Input: dimensioned drawing with shaded views. Units: mm. Origin: part minimum x, y, z. A direction names the side the tool comes from. Give positions to 0.01 mm unless a question says otherwise; leave off trailing zeros. Write each loop counter-clockwise with the first axis right and the second up, starting at its lowest first coordinate (ties: lowest second). Pieces come first, ordered by that corner, then holes. Notation, with made-up numbers: M 87,47 L 119,47 A24 cw 119,74 Z; hole C 25,27 d7. An arc over 180 degrees is marked long. Use CSV: the item, a comma, the result in double quotes. Start each with the question number.
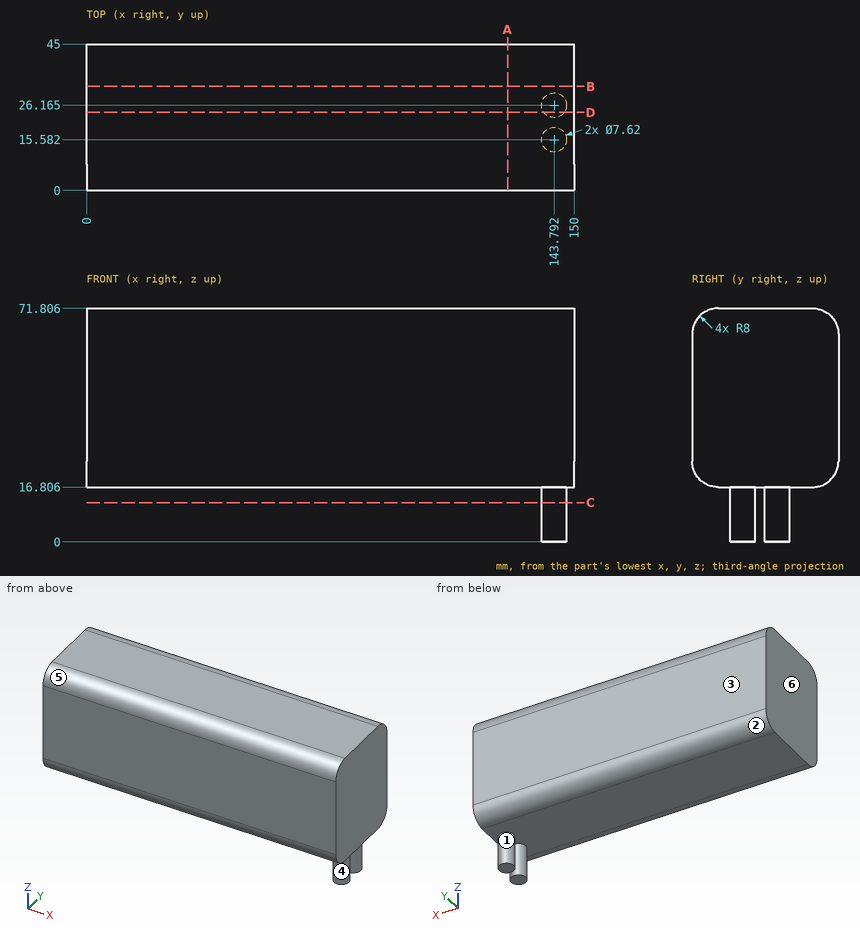
Item 1: Section B-B (y = 32). Return the cut outline in (x, z).
Item 2: Set-up query: the marked faces 1 and 2. Return all of +Z, -Z, +X, -X, +Y, -Y with unobstructed straight access to the full face (end or side cutting, diameter ignored); none if empty.
Item 3: Section A-A (x = 129.5). Return the cut outline in (y, z), plus the area to 3 significant figures.
Item 4: Pull-direction query (Y, two-part tool) for the marked faces 3, 4, 5 and 6; classes: released by +Y, released by -Y, zero draft, split by the parting line, or undercut.
Item 5: Material intervals for probe 1 along Z at (x, y) = (16.5, 9); probe 2 along Y at (x, z) = (12, 64.5); probe 3 along Z at (x, y) = (60.5, 38), sorted ascending.
Item 6: Contact query for flat-ended pins moving along their axis: pin 1 Ø12 at (x, y) = (43, 12.5) entering from -Z; pin 2 Ø3 at (x, z) = (80, 17.5) entering from +Y; pin 3 Ø6 at (x, z) = (23, 21) entering from +Y. Output: stop coordinate, or through.
Item 7: Section C-C (z = 12). Return the cut outline in (x, y) (1 decimal).
Item 8: Section D-D (y = 24). Return the cut outline in (x, z), plus the area to 3 significant figures.
Output values:
1,outline,"M 0,16.81 L 150,16.81 L 150,71.81 L 0,71.81 Z"
2,face 1,"-Z"
2,face 2,"-Z, +X, -X, +Y"
3,outline,"M 0,24.81 A8 ccw 8,16.81 L 37,16.81 A8 ccw 45,24.81 L 45,63.81 A8 ccw 37,71.81 L 8,71.81 A8 ccw 0,63.81 Z"
3,area,"2,420 mm2"
4,face 3,"released by +Y"
4,face 4,"undercut"
4,face 5,"released by -Y"
4,face 6,"zero draft"
5,probe 1,"z = 16.81 to 71.81"
5,probe 2,"y = 0.03 to 44.97"
5,probe 3,"z = 16.87 to 71.74"
6,pin 1,"stops at z = 16.81"
6,pin 2,"stops at y = 42.5"
6,pin 3,"stops at y = 44.96"
7,outline,"C 143.8,15.6 d7.6; C 143.8,26.2 d7.6"
8,outline,"M 0,16.81 L 140.66,16.81 L 140.66,0 L 146.93,0 L 146.93,16.81 L 150,16.81 L 150,71.81 L 0,71.81 Z"
8,area,"8,360 mm2"
